Input: part model. Units: mm. Frame: model coordinates. A direction names the side the tool comes from. Give positions to 0.01 mm unless a question says otherwise; leave off trailing zeros. Write each loop counter-clockwise with the first axis right and the second up, starting at its lowest first coordinate (ties: lowest second). Pieces come first, ordered by that corner, then holes. Notation, with made-up numbers: (21, -24.75) -> (64, -24.75) arc R11 cw to (64, -20.75) -> close; hole circle Ø4 at (-28, 64). An arc over 180 degrees is marked (long way). Return JSON: item names as keys, results as strings. Group by question number.
Item 1: Set-up query: faces 4 (the face through (0, -2, 0)), 5 (the face through (-4.31, 2.29, 10.39)), 6 (the face through (7, 5, -9)). Return all of +Z, -Z, +X, -X, +Y, -Y with unobstructed straight access to the full face (end or side cutting, diameter ignored); none if empty.
Item 2: Section A-A, the plane z = 0. Return loops of the section in (x, y), then the cut area to 4 significant figures.
Item 3: Mould query, pull axis Z, two halves, no side actions, for faces 1 (the face through (3.755, 0.07, 11.923)), 2 (the face through (4.31, -3.48, 10.39)), 3 (the face through (7, -5, -9)). Classes: released by +Z, released by -Z, zero draft, split by the parting line, or undercut.
Item 4: Pin query (flat end, axial travel): P1, Ø2, axis at x = 9, z = -4.5, coming from the +Y side; P2, Ø5, axis at x = -1.5, z = 2, coming from the -Y side; P3, Ø1.5, axis at x = -2.5, y = 0.5, coming from the +Z side. Return the tip coordinate at first contact, or that it passes through.
Item 5: Section D-D, the plane y = -1.5. Return loops of the section in (x, z).
Item 6: Line query: line 1 (X direction, y = 3.15, z = 0); line 2 (Y direction, x = -4.25, z = 0.5); line 3 (X direction, y = 4, z = -4.75). Output: solid intervals per line, ascending. Write a range as [from, to].
Item 7: Section C-C, the plane y = -3.25. Return loops of the section in (x, z).
Item 8: Section B-B, the plane x = 0. Return loops of the section in (y, z).
from build123d import *

# Parameters (mm, degrees)
SKETCH1_R           = 12.5
BOSS_EXTRUDE1_DEPTH = 5
SKETCH2_R           = 11.25
CUT_EXTRUDE1_DEPTH  = 5.5
CUT_EXTRUDE2_START  = -3
SKETCH3_R           = 11.25
CUT_EXTRUDE2_DEPTH  = 3


with BuildPart() as part:
    # Sketch1 → Boss-Extrude1 (new, symmetric)
    with BuildSketch(Plane(origin=(0, 0, 0), x_dir=(1, 0, 0), z_dir=(0, 1, 0))):
        with Locations(Location((0, 0, 0), (0, 0, 270))):
            Circle(SKETCH1_R)
    extrude(amount=BOSS_EXTRUDE1_DEPTH, both=True)

    # Sketch2 → Cut-Extrude1 (cut)
    with BuildSketch(Plane(origin=(0, 5, 0), x_dir=(1, 0, 0), z_dir=(0, 1, 0))):
        with Locations(Location((0, 0, 0), (0, 0, 270))):
            Circle(SKETCH2_R)
    extrude(amount=-CUT_EXTRUDE1_DEPTH, mode=Mode.SUBTRACT)

    # Sketch3 → Cut-Extrude2 (cut)
    with BuildSketch(Plane.XZ.offset(5).offset(CUT_EXTRUDE2_START)):
        with Locations(Location((0, 0, 0), (0, 0, 90))):
            Circle(SKETCH3_R)
    extrude(amount=CUT_EXTRUDE2_DEPTH, mode=Mode.SUBTRACT)


solid = part.part
Answer below:
{
 "1": {"face 4": "-Y", "face 5": "+Y", "face 6": "+Z, -Z, +X, -X, +Y"},
 "2": {"outline": "(-12.5, -5) -> (-11.25, -5) -> (-11.25, -2) -> (11.25, -2) -> (11.25, -5) -> (12.5, -5) -> (12.5, 5) -> (11.25, 5) -> (11.25, -0.5) -> (-11.25, -0.5) -> (-11.25, 5) -> (-12.5, 5) -> close", "area": "58.75 mm2"},
 "3": {"face 1": "split by the parting line", "face 2": "undercut", "face 3": "zero draft"},
 "4": {"P1": "stops at y = -0.5", "P2": "stops at y = -2", "P3": "stops at z = 12.38"},
 "5": {"outline": "circle Ø25 at (0, 0)"},
 "6": {"line 1": "x = [-12.5, -11.25], [11.25, 12.5]", "line 2": "y = [-2, -0.5]", "line 3": "x = [-11.56, -10.2], [10.2, 11.56]"},
 "7": {"outline": "circle Ø25 at (0, 0); hole circle Ø22.5 at (0, 0)"},
 "8": {"outline": "(-5, -12.5) -> (5, -12.5) -> (5, -11.25) -> (-0.5, -11.25) -> (-0.5, 11.25) -> (5, 11.25) -> (5, 12.5) -> (-5, 12.5) -> (-5, 11.25) -> (-2, 11.25) -> (-2, -11.25) -> (-5, -11.25) -> close"}
}
